```python
from build123d import *

# Parameters (mm, degrees)
SKETCH1_W           = 65.278
SKETCH1_H           = 63.754
BOSS_EXTRUDE1_DEPTH = 3.048
SKETCH2_W           = 59.944
SKETCH2_H           = 56.769
BOSS_EXTRUDE2_DEPTH = 3.429
SKETCH3_R           = 1.0668
SKETCH3_R_2         = 0.889
CUT_EXTRUDE1_DEPTH  = 46.751562716
FILLET1_R           = 3.175
SKETCH4_W           = 5.969
SKETCH4_H           = 3.4925
CUT_EXTRUDE2_DEPTH  = 46.751562716
SKETCH5_W           = 49.784
SKETCH5_H           = 4.572
BOSS_EXTRUDE3_DEPTH = 1.5875


with BuildPart() as part:
    # Sketch1 → Boss-Extrude1 (new body)
    with BuildSketch(Plane(origin=(0, 0, 0), x_dir=(1, 0, 0), z_dir=(0, 1, 0))):
        Rectangle(SKETCH1_W, SKETCH1_H)
    extrude(amount=BOSS_EXTRUDE1_DEPTH)

    # Sketch2 → Boss-Extrude2 (add)
    with BuildSketch(Plane(origin=(0, 3.048, 0), x_dir=(1, 0, 0), z_dir=(0, 1, 0))):
        Rectangle(SKETCH2_W, SKETCH2_H)
    extrude(amount=BOSS_EXTRUDE2_DEPTH)

    # Sketch3 → Cut-Extrude1 (cut, through all)
    with BuildSketch(Plane(origin=(0, 3.048, 0), x_dir=(1, 0, 0), z_dir=(0, 1, 0))):
        with Locations(Location((-30, 29.5, 0), (0, 0, 270))):
            Circle(SKETCH3_R)
        with Locations(Location((30, 29.5, 0), (0, 0, 270))):
            Circle(SKETCH3_R)
        with Locations(Location((30, -29.5, 0), (0, 0, 270))):
            Circle(SKETCH3_R_2)
        with Locations(Location((-30, -29.5, 0), (0, 0, 270))):
            Circle(SKETCH3_R_2)
    extrude(amount=-CUT_EXTRUDE1_DEPTH, mode=Mode.SUBTRACT)

    # Fillet1
    fillet1_edges = [part.edges().sort_by_distance(p)[0] for p in [
        (29.972, 4.7625, 28.3845),
        (29.972, 4.7625, -28.3845),
        (-29.972, 4.7625, -28.3845),
        (-29.972, 4.7625, 28.3845),
    ]]
    fillet(fillet1_edges, radius=FILLET1_R)

    # Sketch4 → Cut-Extrude2 (cut, through all)
    with BuildSketch(Plane(origin=(0, 3.048, 0), x_dir=(1, 0, 0), z_dir=(0, 1, 0))):
        with Locations((0, 30.13075)):
            Rectangle(SKETCH4_W, SKETCH4_H)
    extrude(amount=-CUT_EXTRUDE2_DEPTH, mode=Mode.SUBTRACT)

    # Sketch5 → Boss-Extrude3 (add)
    with BuildSketch(Plane.XZ):
        with Locations((0, 34.163)):
            Rectangle(SKETCH5_W, SKETCH5_H)
    extrude(amount=-BOSS_EXTRUDE3_DEPTH)


solid = part.part
```
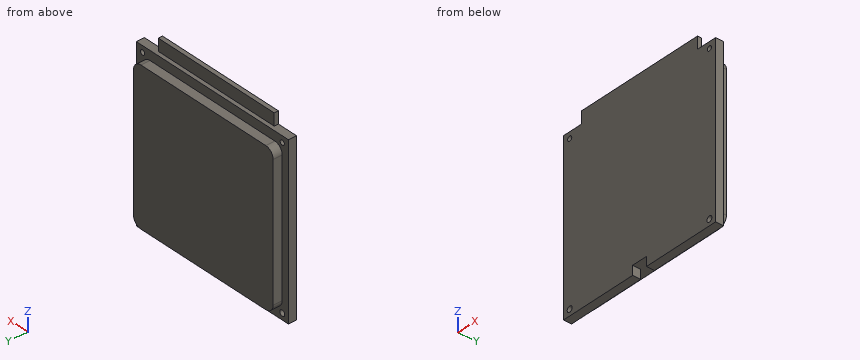
The listing builds one solid part. Answer for the finished solid, in the listing's coordinates (mm). Give positions to 0.01 mm unless a question says otherwise; leave off trailing zeros. Order: outer loops, then holes, each group sorted by start corner. A loop starts at its lowest first (then second) coordinate and runs counter-clockwise, first axis right, second up. Notation, with made-up numbers: M 70,35 L 95,35 A17 ccw 95,43 Z; hole C -34,82 d9. An arc over 180 degrees is marked long. Put each result on its own line as item: value. Start each with the question number.
Item 1: The part is cut by section B-B, the plane z = 29.5. Determine the outline of the cut face in (x, y), and give its area (3 significant figures).
Item 2: The part is cut by section D-D, the plane z = -8.5. Determine the outline of the cut face in (x, y), and give its area (3 significant figures).
Item 3: The part is cut by section A-A, the plane z = -29.5. Determine the outline of the cut face in (x, y), and give its area (3 significant figures).
Item 4: Flat-ended cylindrical pins translate along their axes: P1, Ø1, axis at x = 4, y = 4, coming from the +Z side; P2, Ø1.7, axis at y = 0.5, z = 34, coming from the +X side; P3, Ø0.5, axis at y = 0.5, z = 34, coming from the -X side. Find the tip coordinate at first contact, or state that the pin passes through.
Item 5: Find the intervals of material crossed by line 1 along X through (y, z) = (2, 29.5); line 2 along X through (y, z) = (0.8, -29.5); line 3 along Z through (x, y) = (22, 3.25), in increasing order.
Item 6: The part is cut by section C-C, the plane x = 4.5. Determine the outline of the cut face in (y, z), and give its area (3 significant figures).
Answer key:
1. outline: M -32.64,0 L -30.89,0 L -30.89,3.05 L -32.64,3.05 Z; M -29.11,0 L 29.11,0 L 29.11,3.05 L -29.11,3.05 Z; M 30.89,0 L 32.64,0 L 32.64,3.05 L 30.89,3.05 Z
1. area: 188 mm²
2. outline: M -32.64,0 L 32.64,0 L 32.64,3.05 L 29.97,3.05 L 29.97,6.48 L -29.97,6.48 L -29.97,3.05 L -32.64,3.05 Z
2. area: 405 mm²
3. outline: M -32.64,0 L -31.07,0 L -31.07,3.05 L -32.64,3.05 Z; M -28.93,0 L -2.98,0 L -2.98,3.05 L -28.93,3.05 Z; M 2.98,0 L 28.93,0 L 28.93,3.05 L 2.98,3.05 Z; M 31.07,0 L 32.64,0 L 32.64,3.05 L 31.07,3.05 Z
3. area: 168 mm²
4. P1: stops at z = 28.38
4. P2: stops at x = 24.89
4. P3: stops at x = -24.89
5. line 1: x = -32.64 to -30.89, -29.11 to 29.11, 30.89 to 32.64
5. line 2: x = -32.64 to -31.07, -28.93 to -2.98, 2.98 to 28.93, 31.07 to 32.64
5. line 3: z = -28.38 to 28.38
6. outline: M 0,-31.88 L 3.05,-31.88 L 3.05,-28.38 L 6.48,-28.38 L 6.48,28.38 L 3.05,28.38 L 3.05,31.88 L 1.59,31.88 L 1.59,36.45 L 0,36.45 Z
6. area: 396 mm²
